For this review, take the finished solid that the model builds, in its own axes (mm). Face numbers are marked on the shaded views. A direction names the side the tool comes from. Coordinates: 2 decimals unless noted, no trailing zeros. Write each loop counter-clockwise with the first axis right and the second up, starting at its lowest first coordinate (ties: lowest second). Pieces come first, ordered by that corner, then holes. Notation, with made-up numbers: (88.5, -38.5) -> (108.5, -38.5) arc R3 cw to (108.5, -33.5) -> close; hole circle Ø4 at (75.25, 27.25). An arc over 180 degrees is marked (long way). One line per item, written item: value. Start each with the question number.
1) For pin 1 Ø12.5 at (y, z) = (182, -3.5) entering from -X; pin 2 Ø21 at (x, y) = (-26, 172.5) entering from +Z; pin 3 Ø1.9 at (x, z) = (-34, 1.5) entering from +Y, all flat-tipped, find the tip position at first contact; note any pin that passes through.
2) Add section B-B (y = 184.15). State the section outline as (x, z) points, and give its area (3 significant figures).
3) Add section C-C (y = 37). State the section outline as (x, z) points, and give its area (3 significant figures).
4) Mouldability with a two-part tool opening along X and no side actions: class the marked faces 1, 2, 3 and 4 as released by +X, released by -X, zero draft, split by the parting line, or undercut.
5) Machinability: for the marked faces 5, 6, 7 and 8, which of the approach directions +Z, -Z, +X, -X, +Y, -Y give a long, thin tool a straight path to every point of the face, cutting with its end or side? Answer none if there is none.
6) For probe 1 along X at (y, z) = (29, 0); probe 2 along X at (y, z) = (195, -17); probe 3 along Y at (x, z) = (19.5, -30.5), list the stretches that pass through material, from the lowest coordinate up. Write a range as from..to.
7) Add section A-A (x = 0). State the section outline as (y, z) points, and give its area (3 significant figures).
8) Add section D-D (z = -15). State the section outline as (x, y) points.
from build123d import *

# Parameters (mm, degrees)
SKETCH1_R           = 38.1
BOSS_EXTRUDE1_DEPTH = 152.4
SKETCH2_W           = 63.5
SKETCH2_H           = 42.121134838
BOSS_EXTRUDE2_DEPTH = 63.5
SKETCH3_W           = 25.4
SKETCH3_H           = 42.121134838
CUT_EXTRUDE1_DEPTH  = 63.5
FILLET1_R           = 25.4
SKETCH5_R           = 25.4
CUT_EXTRUDE3_DEPTH  = 50.8
SKETCH4_R           = 12.7
BOSS_EXTRUDE3_DEPTH = 52.578


with BuildPart() as part:
    # Sketch1 → Boss-Extrude1 (new body)
    with BuildSketch(Plane(origin=(0, 0, 0), x_dir=(1, 0, 0), z_dir=(0, 1, 0))):
        with Locations(Location((0, 0, 0), (0, 0, 90))):
            Circle(SKETCH1_R)
    extrude(amount=BOSS_EXTRUDE1_DEPTH)

    # Sketch2 → Boss-Extrude2 (add)
    with BuildSketch(Plane(origin=(0, 152.4, 0), x_dir=(1, 0, 0), z_dir=(0, 1, 0))):
        Rectangle(SKETCH2_W, SKETCH2_H)
    extrude(amount=BOSS_EXTRUDE2_DEPTH)

    # Sketch3 → Cut-Extrude1 (cut)
    with BuildSketch(Plane(origin=(0, 215.9, 0), x_dir=(1, 0, 0), z_dir=(0, 1, 0))):
        Rectangle(SKETCH3_W, SKETCH3_H)
    extrude(amount=-CUT_EXTRUDE1_DEPTH, mode=Mode.SUBTRACT)

    # Fillet1
    # the kernel refuses this fillet: 25.4 mm, written as the material it takes off along each edge
    with BuildSketch(Plane(origin=(50.8, 215.9, -21.060567419), x_dir=(0, -1, 0), z_dir=(-1, 0, 0)), Plane(origin=(-95.25, 215.9, 21.060567419), x_dir=(0, -1, 0), z_dir=(1, 0, 0)), Plane(origin=(95.25, 215.9, -21.060567419), x_dir=(0, -1, 0), z_dir=(-1, 0, 0)), Plane(origin=(-50.8, 215.9, 21.060567419), x_dir=(0, -1, 0), z_dir=(1, 0, 0))) as fillet1_piece_1:
        with BuildLine():
            CenterArc((FILLET1_R, FILLET1_R), FILLET1_R, 180, 90)
            Line((0, FILLET1_R), (0, 0))
            Line((0, 0), (FILLET1_R, 0))
        make_face()
    extrude(amount=146.05, mode=Mode.SUBTRACT)

    # Sketch5 → Cut-Extrude3 (cut)
    with BuildSketch(Plane.XZ):
        with Locations(Location((0, 0, 0), (0, 0, 270))):
            Circle(SKETCH5_R)
    extrude(amount=-CUT_EXTRUDE3_DEPTH, mode=Mode.SUBTRACT)

    # Sketch4 → Boss-Extrude3 (add)
    with BuildSketch(Plane(origin=(31.75, 0, 0), x_dir=(0, 0, -1), z_dir=(1, 0, 0))):
        with Locations((0, 184.15)):
            Circle(SKETCH4_R)
    extrude(amount=-BOSS_EXTRUDE3_DEPTH)


solid = part.part
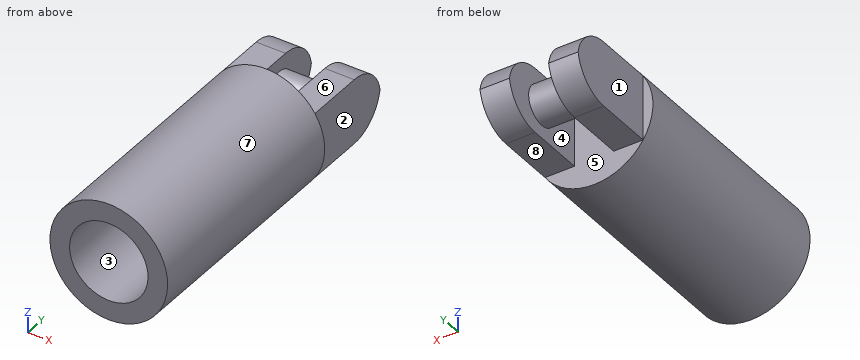
Numbers:
1. pin 1: x = -31.75
1. pin 2: z = 21.06
1. pin 3: y = 152.4
2. outline: (-31.75, -21.06) -> (-12.7, -21.06) -> (-12.7, -12.7) -> (12.7, -12.7) -> (12.7, -21.06) -> (31.75, -21.06) -> (31.75, 21.06) -> (12.7, 21.06) -> (12.7, 12.7) -> (-12.7, 12.7) -> (-12.7, 21.06) -> (-31.75, 21.06) -> close
2. area: 2,250 mm²
3. outline: circle Ø76.2 at (0, 0); hole circle Ø50.8 at (0, 0)
3. area: 2,530 mm²
4. face 1: released by -X
4. face 2: released by +X
4. face 3: undercut
4. face 4: undercut
5. face 5: none
5. face 6: +Z, +X, -X, +Y
5. face 7: +Y, -Y
5. face 8: -Z, +X, -X, +Y
6. probe 1: -38.1..-25.4, 25.4..38.1
6. probe 2: -31.75..-12.7, 12.7..31.75
6. probe 3: 0..152.4
7. outline: (0, -38.1) -> (152.4, -38.1) -> (152.4, 38.1) -> (0, 38.1) -> (0, 25.4) -> (50.8, 25.4) -> (50.8, -25.4) -> (0, -25.4) -> close; circle Ø25.4 at (184.15, 0)
7. area: 9,540 mm²
8. outline: (-35.02, 0) -> (-20.5, 0) -> (-20.5, 50.8) -> (20.5, 50.8) -> (20.5, 0) -> (35.02, 0) -> (35.02, 152.4) -> (31.75, 152.4) -> (31.75, 206.97) -> (12.7, 206.97) -> (12.7, 152.4) -> (-12.7, 152.4) -> (-12.7, 206.97) -> (-31.75, 206.97) -> (-31.75, 152.4) -> (-35.02, 152.4) -> close
